Geometry: final body of the model. Coordinates: model frame, mm. A direction names the side the tool comes from. Give positions to 0.01 mm unless a question says otherwise; leave off trailing zeros. Loops run counter-clockwise (first coordinate to the right, second up) from the corner with the lowest first, then second, coordinate; pieces in that order, holes last.
from build123d import *

# Parameters (mm, degrees)
F0_W     = 21.3086809963
F0_H     = 21.0013445467
F1_DEPTH = 25.4
F3_DEPTH = 53.3642210066


with BuildPart() as f1:
    # F0 (on Right) → F1 (new body)
    with BuildSketch(Plane.YZ):
        with Locations((-10.6543404981, 10.5006722733)):
            Rectangle(F0_W, F0_H)
    extrude(amount=F1_DEPTH)

    # F2 (on face) → F3 (join)
    with BuildSketch(Plane.YZ.offset(25.4)):
        with BuildLine():
            Line((-10.7450820506, 4.6855835698), (-10.7450820506, 17.6185862639))
            ThreePointArc((-10.7450820506, 17.6185862639), (-17.2063226354, 11.1520849168), (-10.7450820506, 4.6855835698))
        make_face()
    extrude(amount=-F3_DEPTH)


solid = f1.part
Item 1: Set-up query: faces 1 (the face through (-13.786, -17.205, 11.294)), 2 (the face through (-14, -10.745, 11)), 3 (the face through (25.4, -11, 11)). Return all of +Z, -Z, +X, -X, +Y, -Y with unobstructed straight access to the full face (end or side cutting, diameter ignored); none if empty.
Values follow:
face 1: -X, -Y
face 2: +Z, -Z, -X, +Y
face 3: +Z, -Z, +X, +Y, -Y
Item 2: Section query B-B on y = -10.25. Return loops of the section in (x, z).
Values follow:
outline: (0, 0) - (25.4, 0) - (25.4, 21) - (0, 21) - close
Item 3: Section query A-A on z = 2.75. Return loops of the section in (x, y).
Values follow:
outline: (0, -21.31) - (25.4, -21.31) - (25.4, 0) - (0, 0) - close
Item 4: Section query D-D on z = 14.5. Return loops of the section in (x, y).
Values follow:
outline: (-27.96, -16.27) - (0, -16.27) - (0, -21.31) - (25.4, -21.31) - (25.4, 0) - (0, 0) - (0, -10.75) - (-27.96, -10.75) - close
Item 5: Ray query, probe 1 along X at (y, z) = (-8.5, 19); probe 2 along Z at (x, y) = (-22.5, -15.75); probe 3 along Y at (x, z) = (-3, 15.25). Return the intervals inside material, ascending.
Values follow:
probe 1: x = 0 to 25.4
probe 2: z = 7.06 to 15.24
probe 3: y = -15.74 to -10.75
Item 6: Pin query (flat end, axial travel): pin 1 (8 mm diameter, centred on x = -5, z = 17.5, fed in from -Y) (3 decimals); pin 2 (1.5 mm diameter, centred on x = -11.5, z = 17.5, fed in from +Y); pin 3 (10 mm diameter, centred on x = -10, z = 4.5, fed in from -Y). Return the tip coordinate at first contact, or that it passes through.
Values follow:
pin 1: stops at y = -16.765
pin 2: stops at y = -10.75
pin 3: stops at y = -16.99
